from build123d import *

# Parameters (mm, degrees)
F0_R     = 15.875
F1_DEPTH = 38.1
F0_R_2   = 9.525
F2_DEPTH = 19.05
F3_R     = 2.54
F4_SIZE  = 2.54


with BuildPart() as f1:
    # F0 (on Front) → F1 (new body)
    with BuildSketch(Plane.XZ):
        with BuildLine():
            ThreePointArc((2.610413, -25.265505), (18.860866, -17.012576), (25.4, 0))
            ThreePointArc((25.4, 0), (18.860866, 17.012576), (2.610413, 25.265505))
            ThreePointArc((2.610413, 25.265505), (-25.4, 0), (2.610413, -25.265505))
        make_face()
        Circle(F0_R, mode=Mode.SUBTRACT)
    extrude(amount=F1_DEPTH)

    # F0 (on Front) → F2 (join)
    with BuildSketch(Plane.XZ):
        with BuildLine():
            ThreePointArc((2.610413, -25.265505), (18.860866, -17.012576), (25.4, 0))
            ThreePointArc((25.4, 0), (18.860866, 17.012576), (2.610413, 25.265505))
            ThreePointArc((2.610413, 25.265505), (-25.4, 0), (2.610413, -25.265505))
        make_face()
        Circle(F0_R, mode=Mode.SUBTRACT)
        with BuildLine():
            ThreePointArc((2.610413, 25.265505), (18.860866, 17.012576), (25.4, 0))
            ThreePointArc((25.4, 0), (18.860866, -17.012576), (2.610413, -25.265505))
            Line((2.610413, -25.265505), (63.744959, -18.949129))
            ThreePointArc((63.744959, -18.949129), (42.737149, 0), (63.744959, 18.949129))
            Line((63.744959, 18.949129), (2.610413, 25.265505))
        make_face()
        with BuildLine():
            ThreePointArc((80.837149, 0), (75.932798, 12.759432), (63.744959, 18.949129))
            ThreePointArc((63.744959, 18.949129), (42.737149, 0), (63.744959, -18.949129))
            ThreePointArc((63.744959, -18.949129), (75.932798, -12.759432), (80.837149, 0))
        make_face()
        with Locations((61.787149, 0)):
            Circle(F0_R_2, mode=Mode.SUBTRACT)
    extrude(amount=F2_DEPTH)

    # F3
    f3_edges = [f1.edges().sort_by_distance(p)[0] for p in [
        (-2.610413, -38.1, 25.265505),
    ]]
    fillet(f3_edges, radius=F3_R)

    # F4
    f4_edges = [f1.edges().sort_by_distance(p)[0] for p in [
        (-15.875, -38.1, 0),
        (52.262149, -19.05, 0),
    ]]
    chamfer(f4_edges, length=F4_SIZE)


solid = f1.part
Here's how the part is built. I have some questions about the finished solid (model axes, mm). Round coordinates to 2 decimals unless told otherwise and drop trailing zeros.
1. Suppose I cut it at B-B (z = -8). State how many separate pieces and enclosed holes the cut face has, and give its area (3 significant figures).
2. Will these pins go through, and if not, where does the flat tip stop? pin 1 Ø12 at (x, y) = (-2, -25.5) entering from -Z; pin 2 Ø3 at (y, z) = (-16, 4.5) entering from -X; pin 3 Ø15 at (x, z) = (61.79, 0) entering from -Y; pin 4 Ø1 at (x, y) = (15, -29) entering from +Z.
3. I need wall thicknesses on L1, parallel to Z at x = 0, y = -6.5 (3 decimals); L2, parallel to Z at x = -10, y = -22.5; L3, parallel to X at y = -11, z = 13.5. Which ranges of each line are inside material? Lowest first, please.
4. If we mould it in two halves opening along Z, with no side actions, what happens to faces 1 (the flat face through (33.606, -9.392, 22.063)), 2 (the flat face through (2, -38.1, 19)), 3 (the conical face through (15.26, -35.683, 4.805))? For each: released by +Z, released by -Z, zero draft, split by the parting line, or undercut.
Answer sheet:
1. separate pieces: 3
1. enclosed holes: 0
1. area: 1,620 mm2
2. pin 1: stops at z = -25.4
2. pin 2: stops at x = -25.22
2. pin 3: passes through
2. pin 4: stops at z = 20.85
3. L1: z = -25.4 to -15.875, 15.875 to 25.4
3. L2: z = -23.35 to -12.33, 12.33 to 23.35
3. L3: x = -21.52 to -8.35, 8.35 to 75.23
4. face 1: released by +Z
4. face 2: zero draft
4. face 3: undercut
